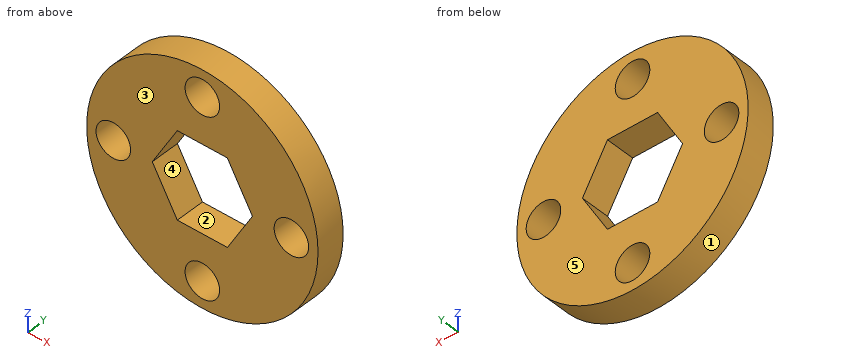
```python
from build123d import *

# Parameters (mm, degrees)
F0_R     = 12.7
F0_R_2   = 1.89865
F1_DEPTH = 3.175


with BuildPart() as f1:
    # F0 (on Front) → F1 (new body)
    with BuildSketch(Plane.XZ):
        Circle(F0_R)
        with Locations((0, -9.779)):
            Circle(F0_R_2, mode=Mode.SUBTRACT)
        with Locations((-9.779, 0)):
            Circle(F0_R_2, mode=Mode.SUBTRACT)
        Polygon((-5.499261, 0), (-2.749631, 4.7625), (2.749631, 4.7625), (5.499261, 0), (2.749631, -4.7625), (-2.749631, -4.7625), align=None, mode=Mode.SUBTRACT)
        with Locations((9.779, 0)):
            Circle(F0_R_2, mode=Mode.SUBTRACT)
        with Locations((0, 9.779)):
            Circle(F0_R_2, mode=Mode.SUBTRACT)
    extrude(amount=F1_DEPTH)


solid = f1.part
```
Input: part model. Units: mm. Frame: model coordinates. Face numbers are marked on the shaded views. A direction names the side the tool comes from. Give positions to 0.01 mm unless a question says otherwise; leave off trailing zeros. Order: outer loops, then holes, each group sorted by start corner. A loop starts at its lowest first (then second) coordinate and runs counter-clockwise, first axis right, second up. Notation, with made-up numbers: (59.25, 50) - (109.25, 50) arc R31 cw to (109.25, 85) - close; hole circle Ø11 at (41, 66). An arc over 180 degrees is marked (long way). Put each result on its own line as item: value.
Item 1: Section query C-C, the plane y = -2.7. Return loops of the section in (x, z), then the cut area to 3 significant figures.
Found:
outline: circle Ø25.4 at (0, 0); hole circle Ø3.8 at (-9.78, 0); hole (-5.5, 0) - (-2.75, -4.76) - (2.75, -4.76) - (5.5, 0) - (2.75, 4.76) - (-2.75, 4.76) - close; hole circle Ø3.8 at (0, -9.78); hole circle Ø3.8 at (0, 9.78); hole circle Ø3.8 at (9.78, 0)
area: 383 mm^2
Item 2: Ray query, L1, parallel to Z at x = 0, y = -1.75; L2, parallel to X at y = -2.7, z = 1.25; L3, parallel to X at y = -1, z = -11. Return the intervals inside material, ascending. Write a range as from..to.
Found:
L1: z = -12.7..-11.68, -7.88..-4.76, 4.76..7.88, 11.68..12.7
L2: x = -12.64..-11.21, -8.35..-4.78, 4.78..8.35, 11.21..12.64
L3: x = -6.35..-1.45, 1.45..6.35
Item 3: Access query for the marked faces 4 and 5. Directions: +Z, -Z, +X, -X, +Y, -Y. A direction counts if a zero-diameter tool reaches every point of the face in a straight line with its end or side. Return the directions, or none.
Found:
face 4: +Y, -Y
face 5: +Z, -Z, +X, -X, +Y
Item 4: Section query D-D, the plane z = 3.5. Return loops of the section in (x, y) (3 decimals), then the cut area to 3 significant figures.
Found:
outline: (-12.208, -3.175) - (-3.479, -3.175) - (-3.479, 0) - (-12.208, 0) - close; (3.479, -3.175) - (12.208, -3.175) - (12.208, 0) - (3.479, 0) - close
area: 55.4 mm^2
Item 5: Contact query for a flat-ended pin moving along its axis: pin 1 (1.5 mm diameter, centred on y = -2.5, z = 8.5, fed in from -X). Output: stop coordinate, or through.
Found:
pin 1: stops at x = -10.06
Item 6: Draft query along X for the marked faces 1, 2 and 3. Return one class per face: +X half, -X half, draft (parallel to the pull), parting line (faces both ways), or undercut.
Found:
face 1: parting line
face 2: undercut
face 3: draft
Item 7: Section query A-A, the plane x = 0. Return loops of the section in (y, z) (1 decimal).
Found:
outline: (-3.2, -12.7) - (0, -12.7) - (0, -11.7) - (-3.2, -11.7) - close; (-3.2, -7.9) - (0, -7.9) - (0, -4.8) - (-3.2, -4.8) - close; (-3.2, 4.8) - (0, 4.8) - (0, 7.9) - (-3.2, 7.9) - close; (-3.2, 11.7) - (0, 11.7) - (0, 12.7) - (-3.2, 12.7) - close
Item 8: Section query B-B, the plane z = -1. Return loops of the section in (x, y) (3 decimals).
Found:
outline: (-12.661, -3.175) - (-11.393, -3.175) - (-11.393, 0) - (-12.661, 0) - close; (-8.165, -3.175) - (-4.922, -3.175) - (-4.922, 0) - (-8.165, 0) - close; (4.922, -3.175) - (8.165, -3.175) - (8.165, 0) - (4.922, 0) - close; (11.393, -3.175) - (12.661, -3.175) - (12.661, 0) - (11.393, 0) - close
